Can you work these out from the model? Positions are in its coordinate system, mm. A direction names the side the tool comes from. Coordinates: 2 decimals unless noted, no trailing zeros. Loops run counter-clockwise (first coordinate to the right, second up) from the corner with the lowest first, then second, coordinate; pieces in that order, holes last.
```python
from build123d import *

# Parameters (mm, degrees)
SKETCH_1_R      = 10.5
EXTRUDE_1_DEPTH = 2


with BuildPart() as part:
    # 草图1 → 凸台-拉伸1 (new body)
    with BuildSketch(Plane.XY):
        with BuildLine():
            Line((-15, 0), (-15, -32.5))
            ThreePointArc((-15, -32.5), (-15.585786438, -33.914213562), (-17, -34.5))
            Line((-17, -34.5), (-19.25, -34.5))
            ThreePointArc((-19.25, -34.5), (-20.664213562, -35.085786438), (-21.25, -36.5))
            Line((-21.25, -36.5), (-21.25, -53.5))
            ThreePointArc((-21.25, -53.5), (-19.931980515, -56.681980515), (-16.75, -58))
            Line((-16.75, -58), (-11.25, -58))
            ThreePointArc((-11.25, -58), (-9.482233047, -57.267766953), (-8.75, -55.5))
            Line((-8.75, -55.5), (-8.75, -55.474127277))
            ThreePointArc((-8.75, -55.474127277), (-8.017766953, -53.706360324), (-6.25, -52.974127277))
            Line((-6.25, -52.974127277), (6.25, -52.974127277))
            ThreePointArc((6.25, -52.974127277), (8.017766953, -53.706360324), (8.75, -55.474127277))
            Line((8.75, -55.474127277), (8.75, -55.5))
            ThreePointArc((8.75, -55.5), (9.482233047, -57.267766953), (11.25, -58))
            Line((11.25, -58), (16.75, -58))
            ThreePointArc((16.75, -58), (19.931980515, -56.681980515), (21.25, -53.5))
            Line((21.25, -53.5), (21.25, -36.5))
            ThreePointArc((21.25, -36.5), (20.664213562, -35.085786438), (19.25, -34.5))
            Line((19.25, -34.5), (17, -34.5))
            ThreePointArc((17, -34.5), (15.585786438, -33.914213562), (15, -32.5))
            Line((15, -32.5), (15, 0))
            ThreePointArc((15, 0), (0, 15), (-15, 0))
        make_face()
        Circle(SKETCH_1_R, mode=Mode.SUBTRACT)
        with BuildLine():
            ThreePointArc((-16.638642988, -49.487063639), (-15, -55), (-13.361357012, -49.487063639))
            ThreePointArc((-13.361357012, -49.487063639), (-12.000091296, -46.997531654), (-13.322348529, -44.487063639))
            ThreePointArc((-13.322348529, -44.487063639), (-15, -39), (-16.677651471, -44.487063639))
            ThreePointArc((-16.677651471, -44.487063639), (-17.999908704, -46.997531654), (-16.638642988, -49.487063639))
        make_face(mode=Mode.SUBTRACT)
        with BuildLine():
            ThreePointArc((-1.704802234, -39.568531819), (-3, -42.037063639), (-1.704802234, -44.505595458))
            ThreePointArc((-1.704802234, -44.505595458), (0, -49.974127277), (1.704802234, -44.505595458))
            ThreePointArc((1.704802234, -44.505595458), (3, -42.037063639), (1.704802234, -39.568531819))
            ThreePointArc((1.704802234, -39.568531819), (0, -34.1), (-1.704802234, -39.568531819))
        make_face(mode=Mode.SUBTRACT)
        with BuildLine():
            ThreePointArc((13.361357012, -49.487063639), (15, -55), (16.638642988, -49.487063639))
            ThreePointArc((16.638642988, -49.487063639), (17.999908704, -46.997531654), (16.677651471, -44.487063639))
            ThreePointArc((16.677651471, -44.487063639), (15, -39), (13.322348529, -44.487063639))
            ThreePointArc((13.322348529, -44.487063639), (12.000091296, -46.997531654), (13.361357012, -49.487063639))
        make_face(mode=Mode.SUBTRACT)
    extrude(amount=EXTRUDE_1_DEPTH)


solid = part.part
```
(1) I want a section at C-C on y = 2. Write out the boundary of the cut face in (x, z), then the cut area to 3 significant figures.
Check values:
outline: (-14.87, 0) - (-10.31, 0) - (-10.31, 2) - (-14.87, 2) - close; (10.31, 0) - (14.87, 0) - (14.87, 2) - (10.31, 2) - close
area: 18.2 mm2
(2) If we mould it in two halves opening along X, with no side actions, what happens to faces 1 (the cylindrical face through (0, 15, 1)), 2 (the flat face through (-15, -16, 1)), 3 (the cylindrical face through (-8.04, -53.73, 0.99))? For each: released by +X, released by -X, zero draft, split by the parting line, or undercut.
Check values:
face 1: split by the parting line
face 2: released by -X
face 3: undercut
(3) I'm going to push flat-ended pins straight in: pin 1 (1 mm diameter, centred on y = -22.5, z = 1, fed in from -X); pin 2 (0.6 mm diameter, centred on x = -18, z = 1, fed in from +Y). Where does each tip first touch, or does it pass through?
Check values:
pin 1: stops at x = -15
pin 2: stops at y = -34.5
(4) I want a section at A-A on y = -52. Write out the boundary of the cut face in (x, z), then the cut area to 3 significant figures.
Check values:
outline: (-21.25, 0) - (-18, 0) - (-18, 2) - (-21.25, 2) - close; (-12, 0) - (12, 0) - (12, 2) - (-12, 2) - close; (18, 0) - (21.25, 0) - (21.25, 2) - (18, 2) - close
area: 61.0 mm2
(5) If I drill on probe 1 along Y at (x, z) = (12.5, 0.4); probe 2 along X at (y, z) = (-42, 1.4); probe 3 along X at (y, z) = (-37.1, 0.55), over which ranges is the centre line in solid material (lowest first)?
Check values:
probe 1: y = -58 to -53.66, -50.34 to -48.63, -45.32 to -43.66, -40.34 to 8.29
probe 2: x = -21.25 to -18, -12 to -3, 3 to 12, 18 to 21.25
probe 3: x = -21.25 to -3, 3 to 21.25
(6) Which directions (+Z, -Z, +X, -X, +Y, -Y) give clear straight access to the entire face, cutting with the end or side of a thin tool? Please do faces 4 (the cylindrical face through (-18, -47, 1)), 5 (the flat face through (15, -16, 1)), 6 (the cylindrical face through (8, -53.69, 0.99)), 7 (the flat face through (-18, -34.5, 1)).
Check values:
face 4: +Z, -Z
face 5: +Z, -Z, +X, +Y
face 6: +Z, -Z, -Y
face 7: +Z, -Z, -X, +Y
(7) I want a section at D-D on y = -42. Write out the boundary of the cut face in (x, z).
Check values:
outline: (-21.25, 0) - (-18, 0) - (-18, 2) - (-21.25, 2) - close; (-12, 0) - (-3, 0) - (-3, 2) - (-12, 2) - close; (3, 0) - (12, 0) - (12, 2) - (3, 2) - close; (18, 0) - (21.25, 0) - (21.25, 2) - (18, 2) - close
(8) I want a section at B-B on x = -7.5. Write out the boundary of the cut face in (y, z).
Check values:
outline: (-53.31, 0) - (-7.35, 0) - (-7.35, 2) - (-53.31, 2) - close; (7.35, 0) - (12.99, 0) - (12.99, 2) - (7.35, 2) - close
